For this review, take the finished solid that the model builds, in its own axes (mm). Give positions to 0.01 mm unless a question says otherwise; leave off trailing zeros. Write each loop counter-clockwise with the first axis right and the second up, starting at its lowest first coordinate (ties: lowest second). Pieces come first, ordered by that corner, then holes.
Q1. Insertion check: P1, Ø4.5, axis at x = 100, y = 46, coming from the +Z side; P2, Ø5, axis at x = -70, y = -46, coming from the +Z side; P3, Ø1.5, axis at x = 259, z = 1.5, coming from the -Y side. Each pin has a flat end and moves straight along its axis. Give the tip position at first contact, or say it passes through.
Q2. For line 1 (X direction, y = 46, z = 0.55); line 2 (X direction, y = -46, z = 0.7); line 3 (Y direction, x = 100, z = 0.7), list the stretches that pass through material, from the lowest coordinate up.
Q3. We need section A-A (z = 2.5). Give the number of separate pieces and of enclosed holes in the cut face, then the cut area to 3 significant figures.
Q4. We need section B-B (y = -5). Write out the cut boundary in (x, z).
```python
from build123d import *

# Parameters (mm, degrees)
SKETCH_1_W          = 550
SKETCH_1_H          = 122
EXTRUDE_1_DEPTH     = 3
CUT_EXTRUDE_2_DEPTH = 282.700195243
SKETCH_2_R          = 2
CUT_EXTRUDE_1_DEPTH = 10
CHAMFER_1_SIZE      = 2


with BuildPart() as part:
    # 草图1 → 凸台-拉伸1 (new body)
    with BuildSketch(Plane.XY):
        Rectangle(SKETCH_1_W, SKETCH_1_H)
    extrude(amount=EXTRUDE_1_DEPTH)

    # 草图3 → 切除-拉伸2 (cut, through all)
    with BuildSketch(Plane.XY.offset(3)):
        Polygon((-275, 31), (-245, 31), (-245, -31), (-227.679491924, -61), (-275, -61), align=None)
        Polygon((245, -31), (227.679491924, -61), (275, -61), (275, 31), (245, 31), align=None)
    extrude(amount=-CUT_EXTRUDE_2_DEPTH, mode=Mode.SUBTRACT)

    # 草图2 → 切除-拉伸1 (cut)
    with BuildSketch(Plane.XY):
        with Locations((-100, 46)):
            Circle(SKETCH_2_R)
        with Locations((-265, 46)):
            Circle(SKETCH_2_R)
        with Locations(Location((265, 46, 0), (0, 0, 180))):
            Circle(SKETCH_2_R)
        with Locations(Location((100, 46, 0), (0, 0, 180))):
            Circle(SKETCH_2_R)
        with Locations((-220, -46)):
            Circle(SKETCH_2_R)
        with Locations((-70, -46)):
            Circle(SKETCH_2_R)
        with Locations(Location((70, -46, 0), (0, 0, 180))):
            Circle(SKETCH_2_R)
        with Locations(Location((220, -46, 0), (0, 0, 180))):
            Circle(SKETCH_2_R)
    extrude(amount=CUT_EXTRUDE_1_DEPTH, mode=Mode.SUBTRACT)

    # 倒角1
    chamfer_1_edges = [part.edges().sort_by_distance(p)[0] for p in [
        (-222, -46, 3),
        (102, 46, 3),
        (267, 46, 3),
        (-267, 46, 3),
        (-72, -46, 3),
        (72, -46, 3),
        (222, -46, 3),
        (-102, 46, 3),
    ]]
    chamfer(chamfer_1_edges, length=CHAMFER_1_SIZE)


solid = part.part
```
Computed:
1. P1: stops at z = 1.25
1. P2: stops at z = 1.5
1. P3: stops at y = 31
2. line 1: x = -275 to -267, -263 to -102, -98 to 98, 102 to 263, 267 to 275
2. line 2: x = -236.34 to -222, -218 to -72, -68 to 68, 72 to 218, 222 to 236.34
2. line 3: y = -61 to 44, 48 to 61
3. separate pieces: 1
3. enclosed holes: 8
3. area: 60,800 mm2
4. outline: (-245, 0) - (245, 0) - (245, 3) - (-245, 3) - close
